from build123d import *

# Parameters (mm, degrees)
SKETCH1_R           = 35
SKETCH1_R_2         = 30
BOSS_EXTRUDE1_DEPTH = 50
SKETCH4_W           = 150
SKETCH4_H           = 10
BOSS_EXTRUDE3_DEPTH = 42
BOSS_EXTRUDE5_START = -6.5
BOSS_EXTRUDE5_DEPTH = 6.5
FILLET1_R           = 16
SKETCH8_W           = 35.5
SKETCH8_H           = 64.245534278
BOSS_EXTRUDE6_DEPTH = 7.5
SKETCH9_W           = 6
SKETCH9_H           = 45
CUT_EXTRUDE1_DEPTH  = 137.330480818
SKETCH10_R          = 7.5
BOSS_EXTRUDE8_DEPTH = 67
CUT_EXTRUDE3_START  = -67
SKETCH12_R          = 30
CUT_EXTRUDE3_DEPTH  = 67
SKETCH13_W          = 3
SKETCH13_H          = 51.427571889
CUT_EXTRUDE4_DEPTH  = 67
SKETCH15_R          = 7.5
CUT_EXTRUDE5_DEPTH  = 113
FILLET2_R           = 6


with BuildPart() as part:
    # Sketch1 → Boss-Extrude1 (new body)
    with BuildSketch(Plane.XY):
        Circle(SKETCH1_R)
        Circle(SKETCH1_R_2, mode=Mode.SUBTRACT)
    extrude(amount=BOSS_EXTRUDE1_DEPTH)



with BuildPart() as body_2:
    # Sketch4 → Boss-Extrude3 (new body)
    with BuildSketch(Plane.XY.offset(2)):
        with Locations((0, -100)):
            Rectangle(SKETCH4_W, SKETCH4_H)
    extrude(amount=BOSS_EXTRUDE3_DEPTH)


with BuildPart() as part_1:
    add(part.part)

    add(body_2.part)  # Boss-Extrude5 merges body 2
    # Sketch5 → Boss-Extrude5 (add)
    with BuildSketch(Plane.XY.offset(44).offset(BOSS_EXTRUDE5_START)):
        with BuildLine():
            Line((-33.5, -10.136567466), (-33.5, -95))
            Line((-33.5, -95), (33.5, -95))
            Line((33.5, -95), (33.5, -10.136567466))
            ThreePointArc((33.5, -10.136567466), (0, -35), (-33.5, -10.136567466))
        make_face()
    extrude(amount=BOSS_EXTRUDE5_DEPTH)

    # Fillet1
    fillet1_edges = [part_1.edges().sort_by_distance(p)[0] for p in [
        (33.5, -95, 40.75),
        (-33.5, -95, 40.75),
    ]]
    fillet(fillet1_edges, radius=FILLET1_R)

    # Sketch8 → Boss-Extrude6 (add, symmetric)
    with BuildSketch(Plane(origin=(0, 0, 0), x_dir=(0, 0, -1), z_dir=(1, 0, 0))):
        with Locations((-19.75, -62.877232861)):
            Rectangle(SKETCH8_W, SKETCH8_H)
    extrude(amount=BOSS_EXTRUDE6_DEPTH, both=True)

    # Sketch9 → Cut-Extrude1 (cut, through all)
    with BuildSketch(Plane.XY.offset(44)):
        with Locations((0, -57.371191548)):
            Rectangle(SKETCH9_W, SKETCH9_H)
    extrude(amount=-CUT_EXTRUDE1_DEPTH, mode=Mode.SUBTRACT)

    # Sketch10 → Boss-Extrude8 (add)
    with BuildSketch(Plane(origin=(33.5, 0, 0), x_dir=(0, 0, -1), z_dir=(1, 0, 0))):
        with BuildLine():
            Line((-44, 42), (-44, 7))
            Line((-44, 7), (-16, 7))
            Line((-16, 7), (-16, 42))
            ThreePointArc((-16, 42), (-30, 56), (-44, 42))
        make_face()
        with Locations((-30, 42)):
            Circle(SKETCH10_R, mode=Mode.SUBTRACT)
    extrude(amount=-BOSS_EXTRUDE8_DEPTH)

    # Sketch12 → Cut-Extrude3 (cut)
    with BuildSketch(Plane.XY.offset(44).offset(CUT_EXTRUDE3_START)):
        Circle(SKETCH12_R)
    extrude(amount=CUT_EXTRUDE3_DEPTH, mode=Mode.SUBTRACT)

    # Sketch13 → Cut-Extrude4 (cut)
    with BuildSketch(Plane.XY.offset(50)):
        with Locations((0, 34.305367012)):
            Rectangle(SKETCH13_W, SKETCH13_H)
    extrude(amount=-CUT_EXTRUDE4_DEPTH, mode=Mode.SUBTRACT)

    # Sketch15 → Cut-Extrude5 (cut)
    with BuildSketch(Plane(origin=(0, 0, 0), x_dir=(1, 0, 0), z_dir=(0, 1, 0))):
        with Locations(Location((-52, -23, 0), (0, 0, 270))):
            Circle(SKETCH15_R)
        with Locations(Location((52, -23, 0), (0, 0, 270))):
            Circle(SKETCH15_R)
    extrude(amount=-CUT_EXTRUDE5_DEPTH, mode=Mode.SUBTRACT)

    # Fillet2
    fillet2_edges = [part_1.edges().sort_by_distance(p)[0] for p in [
        (-75, -100, 2),
        (75, -100, 2),
        (-75, -100, 44),
        (75, -100, 44),
    ]]
    fillet(fillet2_edges, radius=FILLET2_R)


solid = part_1.part
Read the model definition and answer for the solid it produces. Units are mm, in the model's axes. A direction names the side the tool comes from. Round coordinates to 2 decimals unless told otherwise and drop trailing zeros. Order: outer loops, then holes, each group sorted by start corner. A loop starts at its lowest first (then second) coordinate and runs counter-clockwise, first axis right, second up.
1) The part is cut by section B-B on y = -77. Write down the section's boundary in (x, z), plus the area to 3 significant figures.
2) The part is cut by section D-D on x = 52. Write down the section's boundary in (y, z), plus the area to 3 significant figures.
3) Straight lines are drawn through the part: L1, parallel to Z at x = -19, y = 42; L2, parallel to Y at x = 7, z = 27.5; L3, parallel to Y at x = -23.5, z = 30. For each, find the intervals that lie inside material, in ascending order.
4) The part is cut by section C-C on z = 12.5. Write down the section's boundary in (x, y), plus the area to 3 significant figures.
5) For faces 1 (the face through (33.5, -45, 41)), 2 (the face through (7.5, -64, 20)), 3 (the face through (3.25, 34.85, 29.96)), determine the directions among +Z, -Z, +X, -X, +Y, -Y from which every point of the face is accessible in a straight line to the end or side of a thin tool.
6) Flat-ended cylindrical pins translate along their axes: pin 1 (5 mm diameter, centred on y = -52, z = 41, fed in from +X); pin 2 (12 mm diameter, centred on y = -23.5, z = 38, fed in from -X); pin 3 (6 mm diameter, centred on y = -13.5, z = 8.5, fed in from -X). Find the tip coordinate at first contact, or state that the pin passes through.
7) The part is cut by section A-A on x = 19.5. Write down the section's boundary in (y, z), plus the area to 3 significant figures.
8) The mould has two halves that part along X. Classify faces 4 (the face through (-75, -100, 23)), 5 (the face through (73.196, -99.93, 3.711)), 6 (the face through (0, -34.871, 22)): released by +X, released by -X, zero draft, split by the parting line, or undercut.
Resolved:
1. outline: (-33.5, 37.5) - (-7.5, 37.5) - (-7.5, 2) - (-3, 2) - (-3, 44) - (-33.5, 44) - close; (3, 2) - (7.5, 2) - (7.5, 37.5) - (33.5, 37.5) - (33.5, 44) - (3, 44) - close
1. area: 716 mm2
2. outline: (-105, 2) - (-95, 2) - (-95, 15.5) - (-105, 15.5) - close; (-105, 30.5) - (-95, 30.5) - (-95, 44) - (-105, 44) - close
2. area: 270 mm2
3. L1: z = 16 to 22.5, 37.5 to 44
3. L2: y = -105 to -29.17, 29.17 to 34.93, 49.07 to 55.77
3. L3: y = -105 to -95, -25.94 to -18.65, 18.65 to 34.5, 49.5 to 56
4. outline: (-75, -105) - (75, -105) - (75, -95) - (7.5, -95) - (7.5, -34.19) arc R35 ccw to (1.5, 34.97) - (1.5, 29.96) arc R30 cw (long way) to (-1.5, 29.96) - (-1.5, 34.97) arc R35 ccw to (-7.5, -34.19) - (-7.5, -95) - (-75, -95) - close; hole (-3, -79.87) - (3, -79.87) - (3, -34.87) - (-3, -34.87) - close
4. area: 3,140 mm2
5. face 1: +Z, -Z, +X
5. face 2: -Z, +X
5. face 3: +X
6. pin 1: stops at x = 33.5
6. pin 2: stops at x = -33.5
6. pin 3: stops at x = -33.39
7. outline: (-105, 2) - (-95, 2) - (-95, 37.5) - (-29.06, 37.5) - (-29.06, 0) - (-22.8, 0) - (-22.8, 50) - (-29.06, 50) - (-29.06, 44) - (-105, 44) - close; (22.8, 0) - (29.06, 0) - (29.06, 16) - (42, 16) arc R14 ccw to (42, 44) - (29.06, 44) - (29.06, 50) - (22.8, 50) - close; hole circle Ø15 at (42, 30)
7. area: 1,970 mm2
8. face 4: released by -X
8. face 5: released by +X
8. face 6: undercut
